from build123d import *

# Parameters (mm, degrees)
F1_DEPTH = 1000
F2_R     = 1.5


with BuildPart() as f1:
    # F0 (on Front) → F1 (new body)
    with BuildSketch(Plane.XZ):
        Polygon((-7.46, 9.1), (-6.39934, 9.1), (-2.84, 9.1), (-3.74, 10), (-10, 10), (-10, 3.74), (-9.1, 2.84), (-9.1, 6.39934), (-9.1, 7.444134), (-9.124691, 7.46934), (-9.1, 9.1), align=None)
        Polygon((-7.399089, 8.459749), (-6.39934, 7.46), (-6.39934, 9.1), (-7.46, 9.1), (-7.110116, 8.742815), align=None)
        Polygon((-7.46, 6.39934), (-8.470702, 7.410042), (-8.774807, 7.112154), (-9.1, 7.444134), (-9.1, 6.39934), align=None)
        with BuildLine():
            ThreePointArc((-1.917323, 0.856663), (-1.729884, 1.190588), (-1.484924, 1.484924))
            Line((-1.484924, 1.484924), (-7.934896, 7.934896))
            Line((-7.934896, 7.934896), (-8.470702, 7.410042))
            Line((-8.470702, 7.410042), (-7.46, 6.39934))
            Line((-7.46, 6.39934), (-3.90066, 2.84))
            Line((-3.90066, 2.84), (-1.917323, 0.856663))
        make_face()
        with BuildLine():
            ThreePointArc((-1.484924, 1.484924), (-1.190588, 1.729884), (-0.856663, 1.917323))
            Line((-0.856663, 1.917323), (-2.84, 3.90066))
            Line((-2.84, 3.90066), (-6.39934, 7.46))
            Line((-6.39934, 7.46), (-7.399089, 8.459749))
            Line((-7.399089, 8.459749), (-7.934896, 7.934896))
            Line((-7.934896, 7.934896), (-1.484924, 1.484924))
        make_face()
        with BuildLine():
            ThreePointArc((0.856663, 1.917323), (1.484924, 1.484924), (1.917323, 0.856663))
            Line((1.917323, 0.856663), (3.90066, 2.84))
            Line((3.90066, 2.84), (7.46, 6.39934))
            Line((7.46, 6.39934), (9.1, 6.39934))
            Line((9.1, 6.39934), (9.1, 2.84))
            Line((9.1, 2.84), (10, 3.74))
            Line((10, 3.74), (10, 10))
            Line((10, 10), (3.74, 10))
            Line((3.74, 10), (2.84, 9.1))
            Line((2.84, 9.1), (6.39934, 9.1))
            Line((6.39934, 9.1), (6.39934, 7.46))
            Line((6.39934, 7.46), (2.84, 3.90066))
            Line((2.84, 3.90066), (0.856663, 1.917323))
        make_face()
        Polygon((7.112154, 8.774807), (7.46934, 9.124691), (9.1, 9.1), (9.1, 7.46), (8.742815, 7.110116), align=None, mode=Mode.SUBTRACT)
        with BuildLine():
            ThreePointArc((1.917323, 0.856663), (2.053823, 0.437962), (2.1, 0))
            ThreePointArc((2.1, 0), (2.053823, -0.437962), (1.917323, -0.856663))
            Line((1.917323, -0.856663), (3.90066, -2.84))
            Line((3.90066, -2.84), (3.90066, 2.84))
            Line((3.90066, 2.84), (1.917323, 0.856663))
        make_face()
        with BuildLine():
            ThreePointArc((-0.856663, 1.917323), (0, 2.1), (0.856663, 1.917323))
            Line((0.856663, 1.917323), (2.84, 3.90066))
            Line((2.84, 3.90066), (-2.84, 3.90066))
            Line((-2.84, 3.90066), (-0.856663, 1.917323))
        make_face()
        with BuildLine():
            ThreePointArc((-1.917323, -0.856663), (-2.1, 0), (-1.917323, 0.856663))
            Line((-1.917323, 0.856663), (-3.90066, 2.84))
            Line((-3.90066, 2.84), (-3.90066, -2.84))
            Line((-3.90066, -2.84), (-1.917323, -0.856663))
        make_face()
        with BuildLine():
            Line((2.84, -3.90066), (0.856663, -1.917323))
            ThreePointArc((0.856663, -1.917323), (0, -2.1), (-0.856663, -1.917323))
            Line((-0.856663, -1.917323), (-2.84, -3.90066))
            Line((-2.84, -3.90066), (2.84, -3.90066))
        make_face()
        with BuildLine():
            Line((-2.84, -3.90066), (-0.856663, -1.917323))
            ThreePointArc((-0.856663, -1.917323), (-1.190588, -1.729884), (-1.484924, -1.484924))
            Line((-1.484924, -1.484924), (-7.934896, -7.934896))
            Line((-7.934896, -7.934896), (-7.410042, -8.470702))
            Line((-7.410042, -8.470702), (-6.39934, -7.46))
            Line((-6.39934, -7.46), (-2.84, -3.90066))
        make_face()
        with BuildLine():
            Line((-7.934896, -7.934896), (-1.484924, -1.484924))
            ThreePointArc((-1.484924, -1.484924), (-1.729884, -1.190588), (-1.917323, -0.856663))
            Line((-1.917323, -0.856663), (-3.90066, -2.84))
            Line((-3.90066, -2.84), (-7.46, -6.39934))
            Line((-7.46, -6.39934), (-8.459749, -7.399089))
            Line((-8.459749, -7.399089), (-7.934896, -7.934896))
        make_face()
        with BuildLine():
            Line((7.934896, -7.934896), (1.484924, -1.484924))
            ThreePointArc((1.484924, -1.484924), (1.190588, -1.729884), (0.856663, -1.917323))
            Line((0.856663, -1.917323), (2.84, -3.90066))
            Line((2.84, -3.90066), (6.39934, -7.46))
            Line((6.39934, -7.46), (7.399089, -8.459749))
            Line((7.399089, -8.459749), (7.934896, -7.934896))
        make_face()
        with BuildLine():
            Line((3.90066, -2.84), (1.917323, -0.856663))
            ThreePointArc((1.917323, -0.856663), (1.729884, -1.190588), (1.484924, -1.484924))
            Line((1.484924, -1.484924), (7.934896, -7.934896))
            Line((7.934896, -7.934896), (8.470702, -7.410042))
            Line((8.470702, -7.410042), (7.46, -6.39934))
            Line((7.46, -6.39934), (3.90066, -2.84))
        make_face()
        Polygon((9.1, -2.84), (9.1, -6.39934), (9.1, -7.444134), (9.124691, -7.46934), (9.1, -9.1), (7.46, -9.1), (6.39934, -9.1), (2.84, -9.1), (3.74, -10), (10, -10), (10, -3.74), align=None)
        Polygon((9.1, -6.39934), (7.46, -6.39934), (8.470702, -7.410042), (8.774807, -7.112154), (9.1, -7.444134), align=None)
        Polygon((7.110116, -8.742815), (7.399089, -8.459749), (6.39934, -7.46), (6.39934, -9.1), (7.46, -9.1), align=None)
        Polygon((-2.84, -9.1), (-6.39934, -9.1), (-7.444134, -9.1), (-7.46934, -9.124691), (-9.1, -9.1), (-9.1, -7.46), (-9.1, -6.39934), (-9.1, -2.84), (-10, -3.74), (-10, -10), (-3.74, -10), align=None)
        Polygon((-6.39934, -9.1), (-6.39934, -7.46), (-7.410042, -8.470702), (-7.112154, -8.774807), (-7.444134, -9.1), align=None)
        Polygon((-8.742815, -7.110116), (-8.459749, -7.399089), (-7.46, -6.39934), (-9.1, -6.39934), (-9.1, -7.46), align=None)
    extrude(amount=F1_DEPTH)

    # F2
    f2_edges = [f1.edges().sort_by_distance(p)[0] for p in [
        (10, -500, 10),
        (-10, -500, 10),
        (-10, -500, -10),
        (10, -500, -10),
    ]]
    fillet(f2_edges, radius=F2_R)


solid = f1.part
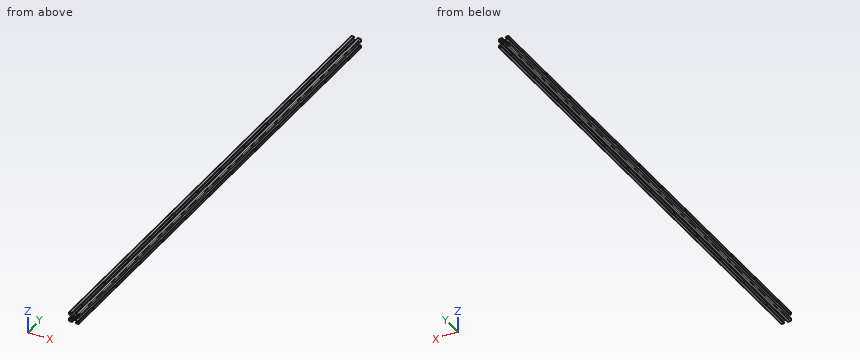
The listing builds one solid part. Answer for the finished solid, in the listing's coordinates (mm). Give positions to 0.01 mm unless a question says otherwise; leave off trailing zeros. One line per question, with ' | ' between items. Start each with the question number.
1. Find the intervals of material crossed by probe 1 along X at (y, z) = (-404, 8); probe 2 along Z at (x, y) = (-7.75, -868.5); probe 3 along X at (y, z) = (-605.5, -3), in increasing order.
2. Given pin 1 Ø6 at (y, z) = (-404.5, 0.5) entering from -X; pin 2 Ø4.5 at (y, z) = (-491.5, 0) entering from +X; pin 3 Ø4.5 at (x, y) = (0, -587.5) entering from -Z, each flat-ended and moving along its own axis, determine where each tip first touches the part or whether it passes through.
3. Section A-A (y = -61.5) is taken. State how many separate pieces and enclosed holes the cut face has, plus the area to 3 significant figures.
Response values:
1) probe 1: -10 to -9.12, -7.87 to -6.4, 6.4 to 7.87, 9.1 to 10 | probe 2: -10 to -9.12, -8.12 to -6.4, 6.4 to 8.12, 9.1 to 10 | probe 3: -9.26 to -9.1, -4.06 to 4.06, 9.1 to 9.26
2) pin 1: x = -9.76 | pin 2: x = 3.9 | pin 3: z = -3.9
3) separate pieces: 1 | enclosed holes: 5 | area: 135 mm2
